```python
from build123d import *

# Parameters (mm, degrees)
F1_DEPTH = 3.175
F2_DEPTH = 5.08
F3_T     = -1.6002
F4_R     = 0.0508


# Not quite as in the source:
# - a feature names something its author has since deleted; it is built from what else it names


with BuildPart() as f1:
    # F0 (on Top) → F1 (new body)
    with BuildSketch(Plane.XY):
        with BuildLine():
            Line((-22.9340831819, 8.5962191019), (-38.8090831819, 8.5962191019))
            Line((-38.8090831819, 8.5962191019), (-38.8090831819, 4.6274691019))
            Line((-38.8090831819, 4.6274691019), (-37.2342831819, 4.6274691019))
            ThreePointArc((-37.2342831819, 4.6274691019), (-34.8466831819, 7.0150691019), (-32.4590831819, 4.6274691019))
            Line((-32.4590831819, 4.6274691019), (-29.2840831819, 4.6274691019))
            ThreePointArc((-29.2840831819, 4.6274691019), (-26.8964831819, 7.0150691019), (-24.5088831819, 4.6274691019))
            Line((-24.5088831819, 4.6274691019), (-22.9340831819, 4.6274691019))
            Line((-22.9340831819, 4.6274691019), (-22.9340831819, 8.5962191019))
        make_face()
        with BuildLine():
            Line((-37.2342831819, 4.6274691019), (-38.8090831819, 4.6274691019))
            Line((-38.8090831819, 4.6274691019), (-38.8090831819, 0.6587191019))
            Line((-38.8090831819, 0.6587191019), (-22.9340831819, 0.6587191019))
            Line((-22.9340831819, 0.6587191019), (-22.9340831819, 4.6274691019))
            Line((-22.9340831819, 4.6274691019), (-24.5088831819, 4.6274691019))
            ThreePointArc((-24.5088831819, 4.6274691019), (-26.8964831819, 2.2398691019), (-29.2840831819, 4.6274691019))
            Line((-29.2840831819, 4.6274691019), (-32.4590831819, 4.6274691019))
            ThreePointArc((-32.4590831819, 4.6274691019), (-34.8466831819, 2.2398691019), (-37.2342831819, 4.6274691019))
        make_face()
        with BuildLine():
            Line((-37.2342831819, -3.3100308981), (-38.8090831819, -3.3100308981))
            Line((-38.8090831819, -3.3100308981), (-38.8090831819, -7.2787808981))
            Line((-38.8090831819, -7.2787808981), (-22.9340831819, -7.2787808981))
            Line((-22.9340831819, -7.2787808981), (-22.9340831819, -3.3100308981))
            Line((-22.9340831819, -3.3100308981), (-24.5088831819, -3.3100308981))
            ThreePointArc((-24.5088831819, -3.3100308981), (-26.8964831819, -5.6976308981), (-29.2840831819, -3.3100308981))
            Line((-29.2840831819, -3.3100308981), (-32.4590831819, -3.3100308981))
            ThreePointArc((-32.4590831819, -3.3100308981), (-34.8466831819, -5.6976308981), (-37.2342831819, -3.3100308981))
        make_face()
        with BuildLine():
            Line((-22.9340831819, 0.6587191019), (-38.8090831819, 0.6587191019))
            Line((-38.8090831819, 0.6587191019), (-38.8090831819, -3.3100308981))
            Line((-38.8090831819, -3.3100308981), (-37.2342831819, -3.3100308981))
            ThreePointArc((-37.2342831819, -3.3100308981), (-34.8466831819, -0.9224308981), (-32.4590831819, -3.3100308981))
            Line((-32.4590831819, -3.3100308981), (-29.2840831819, -3.3100308981))
            ThreePointArc((-29.2840831819, -3.3100308981), (-26.8964831819, -0.9224308981), (-24.5088831819, -3.3100308981))
            Line((-24.5088831819, -3.3100308981), (-22.9340831819, -3.3100308981))
            Line((-22.9340831819, -3.3100308981), (-22.9340831819, 0.6587191019))
        make_face()
    extrude(amount=F1_DEPTH)

    # F0 (on Top) → F2 (join)
    with BuildSketch(Plane.XY):
        with BuildLine():
            Line((-32.4590831819, 4.6274691019), (-37.2342831819, 4.6274691019))
            ThreePointArc((-37.2342831819, 4.6274691019), (-34.8466831819, 2.2398691019), (-32.4590831819, 4.6274691019))
        make_face()
        with BuildLine():
            ThreePointArc((-32.4590831819, 4.6274691019), (-34.8466831819, 7.0150691019), (-37.2342831819, 4.6274691019))
            Line((-37.2342831819, 4.6274691019), (-32.4590831819, 4.6274691019))
        make_face()
        with BuildLine():
            ThreePointArc((-32.4590831819, -3.3100308981), (-34.8466831819, -0.9224308981), (-37.2342831819, -3.3100308981))
            Line((-37.2342831819, -3.3100308981), (-32.4590831819, -3.3100308981))
        make_face()
        with BuildLine():
            Line((-32.4590831819, -3.3100308981), (-37.2342831819, -3.3100308981))
            ThreePointArc((-37.2342831819, -3.3100308981), (-34.8466831819, -5.6976308981), (-32.4590831819, -3.3100308981))
        make_face()
        with BuildLine():
            ThreePointArc((-29.2840831819, -3.3100308981), (-26.8964831819, -5.6976308981), (-24.5088831819, -3.3100308981))
            Line((-24.5088831819, -3.3100308981), (-29.2840831819, -3.3100308981))
        make_face()
        with BuildLine():
            Line((-29.2840831819, -3.3100308981), (-24.5088831819, -3.3100308981))
            ThreePointArc((-24.5088831819, -3.3100308981), (-26.8964831819, -0.9224308981), (-29.2840831819, -3.3100308981))
        make_face()
        with BuildLine():
            ThreePointArc((-29.2840831819, 4.6274691019), (-26.8964831819, 2.2398691019), (-24.5088831819, 4.6274691019))
            Line((-24.5088831819, 4.6274691019), (-29.2840831819, 4.6274691019))
        make_face()
        with BuildLine():
            Line((-29.2840831819, 4.6274691019), (-24.5088831819, 4.6274691019))
            ThreePointArc((-24.5088831819, 4.6274691019), (-26.8964831819, 7.0150691019), (-29.2840831819, 4.6274691019))
        make_face()
    extrude(amount=F2_DEPTH)

    # F3
    f3_openings = [f1.faces().sort_by_distance(p)[0] for p in [
        (-30.871583, 0.658719, 0),
    ]]
    offset(amount=F3_T, openings=f3_openings, kind=Kind.INTERSECTION)

    # F4
    f4_edges = [f1.edges().sort_by_distance(p)[0] for p in [
        (-32.459083, -3.310031, 5.08),
        (-29.284083, -3.310031, 5.08),
        (-29.284083, 4.627469, 5.08),
        (-37.234283, 4.627469, 5.08),
    ]]
    fillet(f4_edges, radius=F4_R)


solid = f1.part
```
Check sheet for the modelled part. Datum: model origin and axes. Units: mm. A direction names the side the tool comes from. Give positions to 0.01 mm unless a question says otherwise; leave off trailing zeros. Loops run counter-clockwise (first coordinate to the right, second up) from the corner with the lowest first, then second, coordinate; pieces in that order, holes last. Notation, with made-up numbers: (-22.75, 65) - (3.25, 65) arc R22 ccw to (3.25, 94) - close; hole circle Ø10 at (-17.75, 56.25). An arc over 180 degrees is marked (long way). One line per question, with ' | ' between items. Start each with the question number.
1. Gauge pin test, flat ends, axial feed: pin 1 Ø0.5 at (x, y) = (-35, -3) entering from -Z; pin 2 Ø2.5 at (x, y) = (-26.9, 4.63) entering from -Z. Record the tip position at first contact, or that the pin passes through.
2. Set-up check for faces 1 (the cylindrical face through (-32.95, -1.86, 4.09)), 2 (the flat face through (-27, -3, 5.08)), 3 (the flat face through (-24.534, 1, 1)): record each of +Z, -Z, +X, -X, +Y, -Y from which the full face is reachable in a straight line by a thin tool's end or side.
3. Cross-section at C-C, the plane x = -32. Enter the section's corners in (y, z) (3 decimals).
4. Cross-section at A-A, the plane z = 0.95. Enter the section's corners in (x, y).
5. Cross-section at D-D, the plane z = 2.3. Enter the section's corners in (x, y), plus the area to 3 significant figures.
6. Draft check along X on faces 4 (the flat face through (-27, 5, 5.08)), 5 (the flat face through (-35, 5, 3.48)), 6 (the flat face through (-38.809, 1, 2)), 7 (the cylindrical face through (-34.119, 4.326, 2.514)). Enter one of: released by +X, released by -X, zero draft, split by the parting line, or undercut.
7. Cross-section at B-B, the plane y = 1.5. Enter the section's corners in (x, z) (3 decimals).
8. Material ranges on line 1 along X through (y, z) = (-4.5, 1.15); line 2 along Y through (x, z) = (-26.5, 1.45); line 3 along Z through (x, y) = (-37.75, -4) (3 decimals), recorded low to high. Write a range as [from, to].
Check result:
1) pin 1: stops at z = 3.48 | pin 2: stops at z = 1.57
2) face 1: +Z | face 2: +Z, +X, -X, +Y, -Y | face 3: -Z
3) outline: (-7.279, 0) - (-5.679, 0) - (-5.679, 1.575) - (6.996, 1.575) - (6.996, 0) - (8.596, 0) - (8.596, 3.175) - (-7.279, 3.175) - close
4) outline: (-38.81, -7.28) - (-22.93, -7.28) - (-22.93, 8.6) - (-38.81, 8.6) - close; hole (-37.21, -5.68) - (-24.53, -5.68) - (-24.53, 7) - (-37.21, 7) - close
5) outline: (-38.81, -7.28) - (-22.93, -7.28) - (-22.93, 8.6) - (-38.81, 8.6) - close; hole circle Ø1.57 at (-34.85, -3.31); hole circle Ø1.57 at (-34.85, 4.63); hole circle Ø1.57 at (-26.9, -3.31); hole circle Ø1.57 at (-26.9, 4.63) | area: 244 mm2
6) face 4: zero draft | face 5: undercut | face 6: released by -X | face 7: undercut
7) outline: (-38.809, 0) - (-37.209, 0) - (-37.209, 1.575) - (-24.534, 1.575) - (-24.534, 0) - (-22.934, 0) - (-22.934, 3.175) - (-38.809, 3.175) - close
8) line 1: x = [-38.81, -37.21], [-24.53, -22.93] | line 2: y = [-7.28, -5.68], [7, 8.6] | line 3: z = [0, 3.175]
